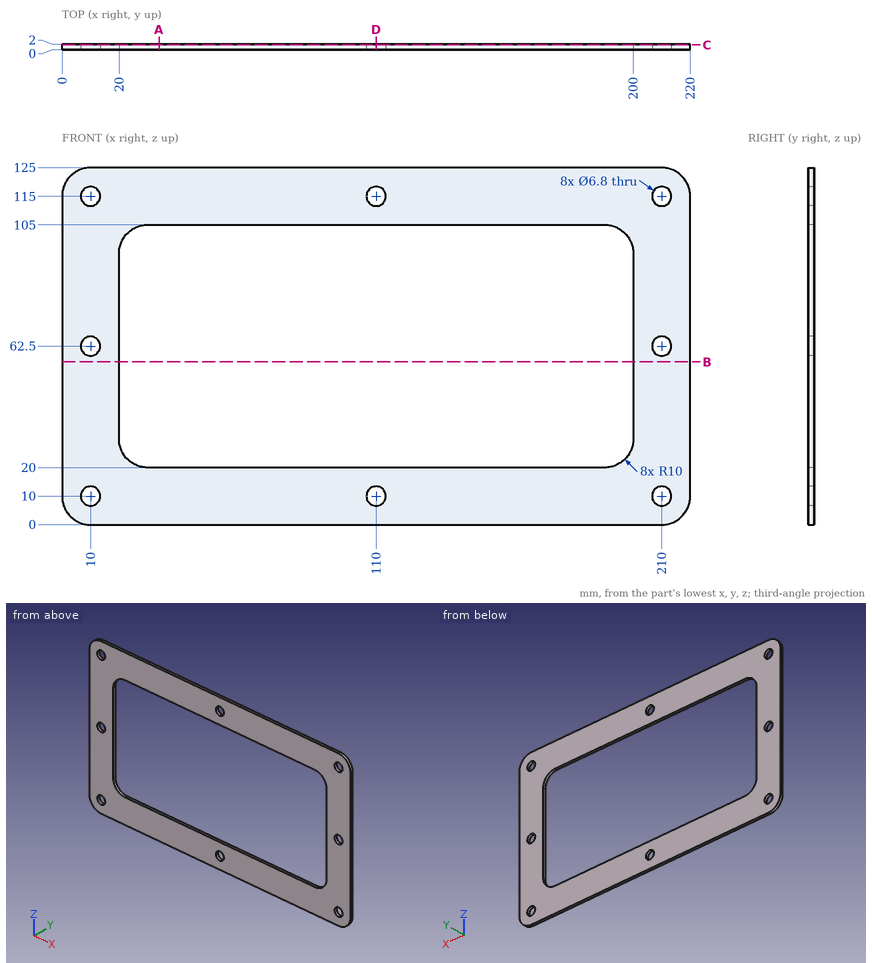
Verification items for this drawing (mm, ordinates from the low corner). Coordinates: 2 decimals unless noted, no trailing zeros. Loops run counter-clockwise (first coordinate to the right, second up) from the corner with the lowest first, then second, coordinate; pieces in that order, holes last. Notation, with made-up numbers: (66, -38.5) - (115, -38.5) arc R34 ccw to (115, -7.5) - close; hole circle Ø4 at (23.5, 72.25). An arc over 180 degrees is marked (long way). Answer as a JSON object with one key per item and string values.
(1) Cross-section at C-C, the plane y = 1.7. Count the separate pieces of the cut face and the enclosed holes in it, then the cut area to 3 significant figures.
Response:
{"separate pieces": "1", "enclosed holes": "9", "area": "11,900 mm²"}
(2) Cross-section at A-A, the plane x = 34. Record the boundary of the cut face in (y, z).
Response:
{"outline": "(0, 0) - (2, 0) - (2, 20) - (0, 20) - close; (0, 105) - (2, 105) - (2, 125) - (0, 125) - close"}
(3) Scan lines: line 1 along Z through (x, y) = (110, 1.35); line 2 along X through (y, z) = (1.2, 115); line 3 along X through (y, z) = (1.6, 41.5). Record each from-to range of solid material in increasing order.
Response:
{"line 1": "z = 0 to 6.6, 13.4 to 20, 105 to 111.6, 118.4 to 125", "line 2": "x = 0 to 6.6, 13.4 to 106.6, 113.4 to 206.6, 213.4 to 220", "line 3": "x = 0 to 20, 200 to 220"}
(4) Cross-section at D-D, the plane x = 110. Record the boundary of the cut face in (y, z), then the cut area to 3 significant figures.
Response:
{"outline": "(0, 0) - (2, 0) - (2, 6.6) - (0, 6.6) - close; (0, 13.4) - (2, 13.4) - (2, 20) - (0, 20) - close; (0, 105) - (2, 105) - (2, 111.6) - (0, 111.6) - close; (0, 118.4) - (2, 118.4) - (2, 125) - (0, 125) - close", "area": "52.8 mm²"}
(5) Cross-section at B-B, the plane z = 57. Record the boundary of the cut face in (x, y), then the cut area to 3 significant figures.
Response:
{"outline": "(0, 0) - (20, 0) - (20, 2) - (0, 2) - close; (200, 0) - (220, 0) - (220, 2) - (200, 2) - close", "area": "80.0 mm²"}
